Source: CAD feature listing. Evaluate the final solid. Frame: model axes, mm. A direction names the side the tool comes from. Round coordinates to 2 decimals unless told otherwise and drop trailing zeros. Order: outer loops, then holes, each group sorted by start corner. A loop starts at its lowest first (then second) coordinate and runs counter-clockwise, first axis right, second up.
```python
from build123d import *

# Parameters (mm, degrees)
SKETCH1_W               = 60
SKETCH1_H               = 60
BOSS_EXTRUDE1_DEPTH     = 10
BOSS_EXTRUDE2_DEPTH     = 10
SKETCH3_R               = 10
CUT_EXTRUDE1_DEPTH      = 44.588989435
SKETCH4_R               = 3.15
CUT_EXTRUDE2_DEPTH      = 44.588989435
SKETCH5_W               = 10
SKETCH5_H               = 15
BOSS_EXTRUDE3_DEPTH     = 45
BOSS_EXTRUDE4_START     = 5
SKETCH6_R               = 10
BOSS_EXTRUDE4_DEPTH     = 5
CUT_EXTRUDE4_REACH      = 87
CUT_EXTRUDE4_END_RADIUS = 22.5
SKETCH7_R               = 1.65
SKETCH8_W               = 11.7
SKETCH8_H               = 15
BOSS_EXTRUDE5_DEPTH     = 10
SKETCH9_W               = 16.7
SKETCH9_H               = 10
CUT_EXTRUDE5_DEPTH      = 71.931304796
CUT_EXTRUDE6_REACH      = 85.258
SKETCH11_R              = 2
SKETCH12_W              = 10
SKETCH12_H              = 15
CUT_EXTRUDE7_DEPTH      = 10
SKETCH15_R              = 1.65
CUT_EXTRUDE8_DEPTH      = 10
LPATTERN1_COUNT         = 3
LPATTERN1_PITCH         = 10
SKETCH16_W              = 100
SKETCH16_H              = 40
BOSS_EXTRUDE6_DEPTH     = 10
SKETCH17_R              = 1.65
CUT_EXTRUDE9_DEPTH      = 106


with BuildPart() as part:
    # Sketch1 → Boss-Extrude1 (new body)
    with BuildSketch(Plane.XY):
        Rectangle(SKETCH1_W, SKETCH1_H)
    extrude(amount=BOSS_EXTRUDE1_DEPTH)

    # Sketch2 → Boss-Extrude2 (add)
    with BuildSketch(Plane.XY.offset(10)):
        with BuildLine():
            Line((-11.25, 19.485571585), (-12.5, 21.650635095))
            ThreePointArc((-12.5, 21.650635095), (-24.850399784, -2.730866272), (-7.5, -23.848480035))
            Line((-7.5, -23.848480035), (-7.5, -30))
            Line((-7.5, -30), (7.5, -30))
            Line((7.5, -30), (7.5, -23.848480035))
            ThreePointArc((7.5, -23.848480035), (24.850399784, -2.730866272), (12.5, 21.650635095))
            Line((12.5, 21.650635095), (11.25, 19.485571585))
            ThreePointArc((11.25, 19.485571585), (0, -22.5), (-11.25, 19.485571585))
        make_face()
    extrude(amount=BOSS_EXTRUDE2_DEPTH)

    # Sketch3 → Cut-Extrude1 (cut, through all)
    with BuildSketch(Plane.XY.offset(10)):
        Circle(SKETCH3_R)
    extrude(amount=-CUT_EXTRUDE1_DEPTH, mode=Mode.SUBTRACT)

    # Sketch4 → Cut-Extrude2 (cut, through all)
    with BuildSketch(Plane.XY.offset(10)):
        with Locations((-25, 25)):
            Circle(SKETCH4_R)
        with Locations((25, 25)):
            Circle(SKETCH4_R)
        with Locations((25, -25)):
            Circle(SKETCH4_R)
        with Locations((-25, -25)):
            Circle(SKETCH4_R)
    extrude(amount=-CUT_EXTRUDE2_DEPTH, mode=Mode.SUBTRACT)

    # Sketch5 → Boss-Extrude3 (add)
    with BuildSketch(Plane(origin=(0, 0, 0), x_dir=(-1, 0, 0), z_dir=(0, 0, -1))):
        with Locations((35, 0)):
            Rectangle(SKETCH5_W, SKETCH5_H)
    boss_extrude3 = extrude(amount=-BOSS_EXTRUDE3_DEPTH)

    # Mirror1: Boss-Extrude3 across plane
    add(boss_extrude3.mirror(Plane.ZY))

    # Sketch6 → Boss-Extrude4 (add)
    with BuildSketch(Plane.XY.offset(30).offset(BOSS_EXTRUDE4_START)):
        with BuildLine():
            Line((30, 7.5), (12.990381057, 7.5))
            ThreePointArc((12.990381057, 7.5), (0, 15), (-12.990381057, 7.5))
            Line((-12.990381057, 7.5), (-30, 7.5))
            Line((-30, 7.5), (-30, -7.5))
            Line((-30, -7.5), (-12.990381057, -7.5))
            ThreePointArc((-12.990381057, -7.5), (0, -15), (12.990381057, -7.5))
            Line((12.990381057, -7.5), (30, -7.5))
            Line((30, -7.5), (30, 7.5))
        make_face()
        Circle(SKETCH6_R, mode=Mode.SUBTRACT)
    extrude(amount=-BOSS_EXTRUDE4_DEPTH)

    # Cut-Extrude4: up to this cylinder (the profile starts outside it)
    cut_extrude4_end = Plane(origin=(0, 0, 15), z_dir=(0, 0, -1)) * Cylinder(CUT_EXTRUDE4_END_RADIUS, 220, mode=Mode.PRIVATE)
    # Sketch7 → Cut-Extrude4 (cut, up to the surface)
    with BuildSketch(Plane(origin=(0, -30, 0), x_dir=(-1, 0, 0), z_dir=(0, -1, 0)), mode=Mode.PRIVATE) as cut_extrude4_sk1:
        with Locations(Location((0, -15, 0), (0, 0, 90))):
            Circle(SKETCH7_R)
    cut_extrude4_tool1 = extrude(cut_extrude4_sk1.sketch, amount=-CUT_EXTRUDE4_REACH, mode=Mode.PRIVATE) - cut_extrude4_end
    add(cut_extrude4_tool1.solids().sort_by_distance((0, -30, 15))[0], mode=Mode.SUBTRACT)

    # Sketch8 → Boss-Extrude5 (add)
    with BuildSketch(Plane.XY.offset(35)):
        with Locations((-24.15, 0)):
            Rectangle(SKETCH8_W, SKETCH8_H)
    extrude(amount=BOSS_EXTRUDE5_DEPTH)

    # Sketch9 → Cut-Extrude5 (cut, through all)
    with BuildSketch(Plane.XZ.offset(7.5)):
        with Locations((-31.65, 40)):
            Rectangle(SKETCH9_W, SKETCH9_H)
    extrude(amount=-CUT_EXTRUDE5_DEPTH, mode=Mode.SUBTRACT)

    # Sketch11 → Cut-Extrude6 (cut, up to next)
    with BuildSketch(Plane.ZY.offset(23.3), mode=Mode.PRIVATE) as cut_extrude6_sk1:
        with Locations((40, 0)):
            Circle(SKETCH11_R)
    cut_extrude6_tool1 = extrude(cut_extrude6_sk1.sketch, amount=-CUT_EXTRUDE6_REACH, mode=Mode.PRIVATE) & part.part
    add(cut_extrude6_tool1.solids().sort_by_distance((-23.3, 0, 40))[0], mode=Mode.SUBTRACT)

    # Sketch12 → Cut-Extrude7 (cut)
    with BuildSketch(Plane.ZY.offset(-30)):
        with Locations((40, 0)):
            Rectangle(SKETCH12_W, SKETCH12_H)
    extrude(amount=-CUT_EXTRUDE7_DEPTH, mode=Mode.SUBTRACT)

    # Sketch15 → Cut-Extrude8 (cut)
    with BuildSketch(Plane.ZY.offset(40)):
        with Locations(Location((5, 0, 0), (0, 0, 270))):
            Circle(SKETCH15_R)
    cut_extrude8 = extrude(amount=-CUT_EXTRUDE8_DEPTH, mode=Mode.SUBTRACT)

    # LPattern1: Cut-Extrude8 ×3
    with Locations(*[(0, 0, i * LPATTERN1_PITCH) for i in range(1, LPATTERN1_COUNT)]):
        add(cut_extrude8, mode=Mode.SUBTRACT)

    # Sketch16 → Boss-Extrude6 (add)
    with BuildSketch(Plane(origin=(0, 0, 0), x_dir=(-1, 0, 0), z_dir=(0, 0, -1))):
        with Locations((-20, 50)):
            Rectangle(SKETCH16_W, SKETCH16_H)
    extrude(amount=-BOSS_EXTRUDE6_DEPTH)

    # Sketch17 → Cut-Extrude9 (cut, through all)
    with BuildSketch(Plane.XY.offset(10)):
        with Locations((66, 34)):
            Circle(SKETCH17_R)
        with Locations((66, 66)):
            Circle(SKETCH17_R)
        with Locations((34, 66)):
            Circle(SKETCH17_R)
        with Locations((34, 34)):
            Circle(SKETCH17_R)
    extrude(amount=-CUT_EXTRUDE9_DEPTH, mode=Mode.SUBTRACT)


solid = part.part
```
1. Line query: line 1 along Y through (x, z) = (-19.8, 40); line 2 along Z through (x, y) = (-13.5, 3); line 3 along Z through (x, y) = (0, -24). Output: solid intervals per line, ascending.
2. Section B-B on x = 66. Return loops of the section in (y, z), plus the area to 3 significant figures.
3. Access query for faces 4 (the face through (-30, -19, 5)), 5 (the face through (32, 7.5, 21)), 6 (the face through (-23.3, -2, 41)), 7 (the face through (-35.1, 0.4, 3.4)), 8 (the face through (-7.5, -27, 15)). Directions: +Z, -Z, +X, -X, +Y, -Y. A direction counts if a zero-diameter tool reaches every point of the face in a straight line with its end or side. Return the directions, or none.
4. Pull-direction query (Y, two-part tool) for faces 1 (the face through (7.5, -27, 15)), 2 (the face through (-30, 0, 5)), 3 (the face through (-32, -7.5, 22)); classes: released by +Y, released by -Y, zero draft, split by the parting line, or undercut.
5. Section A-A on z = 40. Return loops of the section in (x, y), plus the area to 3 significant figures.
6. First-contact query: pin 1 (5 mm diameter, centred on x = -25, y = 25, fed in from +Z); pin 2 (12 mm diameter, centred on x = -29.5, y = 0, fed in from +Z); pin 3 (3 mm diameter, centred on y = 6, z = 11.5, fed in from +X); pin 4 (2 mm diameter, centred on x = 12, z = 31.5, fed in from +Y). Flat tips, straight axial feed; report the tip coordinate or a pass-through.
7. Section D-D on z = 5. State how many separate pieces and enclosed holes the cut face has, plus the area to 3 significant figures.
8. Section C-C on y = 25. Return loops of the section in (x, z).
Result:
1. line 1: y = -7.5 to -2, 2 to 7.5
1. line 2: z = 0 to 10, 30 to 35
1. line 3: z = 0 to 13.35, 16.65 to 20
2. outline: (30, 0) - (32.35, 0) - (32.35, 10) - (30, 10) - close; (35.65, 0) - (64.35, 0) - (64.35, 10) - (35.65, 10) - close; (67.65, 0) - (70, 0) - (70, 10) - (67.65, 10) - close
2. area: 334 mm2
3. face 4: +Z, -Z, -X, -Y
3. face 5: +Z, +X
3. face 6: +Z, -X, +Y, -Y
3. face 7: -X
3. face 8: +Z, -X, -Y
4. face 1: zero draft
4. face 2: undercut
4. face 3: released by -Y
5. outline: (-23.3, -7.5) - (-18.3, -7.5) - (-18.3, -2) - (-23.3, -2) - close; (-23.3, 2) - (-18.3, 2) - (-18.3, 7.5) - (-23.3, 7.5) - close
5. area: 55.0 mm2
6. pin 1: passes through
6. pin 2: stops at z = 35
6. pin 3: stops at x = 40
6. pin 4: stops at y = 10.2
7. separate pieces: 1
7. enclosed holes: 9
7. area: 7,390 mm2
8. outline: (-30, 0) - (-28.15, 0) - (-28.15, 10) - (-30, 10) - close; (-21.85, 0) - (21.85, 0) - (21.85, 10) - (-21.85, 10) - close; (28.15, 0) - (30, 0) - (30, 10) - (28.15, 10) - close
